```python
from build123d import *

# Parameters (mm, degrees)
BOSS_EXTRUDE1_DEPTH      = 37.5
BOSS_EXTRUDE1_DEPTH_BACK = 37.5
SKETCH1_W                = 20
SKETCH1_H                = 10
SKETCH3_W                = 20
SKETCH3_H                = 5
BOSS_EXTRUDE2_DEPTH      = 20
FILLET1_R                = 10
SKETCH4_R                = 2.75
CUT_EXTRUDE1_DEPTH       = 59.84301148
FILLET1_OF_MIRROR3_R     = 10
CHAMFER1_SIZE            = 8.660254038
CHAMFER1_SIZE_2          = 5
SKETCH6_R                = 8.5
CUT_EXTRUDE2_DEPTH       = 5
CUT_EXTRUDE3_DEPTH       = 59.576872569
CUT_EXTRUDE3_DEPTH_BACK  = 59.576872569
SKETCH7_R                = 2


# Some blends are built 0.0001 mm under size
with BuildPart() as part:
    # Sketch1 → Boss-Extrude1 (new, two sides: drawn at the far end of the back side and taken through both)
    with BuildSketch(Plane.XY.offset(-BOSS_EXTRUDE1_DEPTH_BACK)):
        Rectangle(SKETCH1_W, SKETCH1_H)
    extrude(amount=BOSS_EXTRUDE1_DEPTH + BOSS_EXTRUDE1_DEPTH_BACK)

    # Sketch3 → Boss-Extrude2 (add)
    with BuildSketch(Plane(origin=(0, 0, -37.5), x_dir=(-1, 0, 0), z_dir=(0, 0, -1))):
        Rectangle(SKETCH3_W, SKETCH3_H)
    boss_extrude2 = extrude(amount=BOSS_EXTRUDE2_DEPTH)

    # Fillet1
    fillet1_edges = [part.edges().sort_by_distance(p)[0] for p in [
        (-10, 0, -57.5),
        (10, 0, -57.5),
    ]]
    fillet(fillet1_edges, radius=FILLET1_R - 0.0001)  # a hair under: the kernel refuses the full size

    # Sketch4 → Cut-Extrude1 (cut, through all)
    with BuildSketch(Plane(origin=(0, 2.5, 0), x_dir=(1, 0, 0), z_dir=(0, 1, 0))):
        with Locations(Location((0, 47.5, 0), (0, 0, 270))):
            Circle(SKETCH4_R)
    cut_extrude1 = extrude(amount=-CUT_EXTRUDE1_DEPTH, mode=Mode.SUBTRACT)

    # Mirror3: Boss-Extrude2, Cut-Extrude1 across plane
    add(boss_extrude2.mirror(Plane.XY))
    add(cut_extrude1.mirror(Plane.XY), mode=Mode.SUBTRACT)

    # Fillet1 of Mirror3
    fillet1_of_mirror3_edges = [part.edges().sort_by_distance(p)[0] for p in [
        (-10, 0, 57.5),
        (10, 0, 57.5),
    ]]
    fillet(fillet1_of_mirror3_edges, radius=FILLET1_OF_MIRROR3_R - 0.0001)  # a hair under: the kernel refuses the full size

    # Chamfer1
    # the kernel refuses this chamfer: 8.660254038, 5 mm, written as the material it takes off along each edge
    with BuildSketch(Plane(origin=(32.404819853, 5, -37.5), x_dir=(0, 0.019326765612700598, 0.9998132206222078), z_dir=(-1, 0, 0))) as chamfer1_piece_1_section:
        Polygon((CHAMFER1_SIZE * 0.999813220604, -CHAMFER1_SIZE * 0.0193267656124), (-CHAMFER1_SIZE_2 * 0.0193267656127, -CHAMFER1_SIZE_2 * 0.999813220622), (0, 0), align=None)
    chamfer1_piece_1 = extrude(amount=64.809639706, mode=Mode.PRIVATE)
    chamfer1_piece_1 = split(chamfer1_piece_1, bisect_by=Plane(origin=(0, 2.5, -34.039331058), z_dir=(0, 1, 0)), keep=Keep.TOP, mode=Mode.PRIVATE)
    add(chamfer1_piece_1, mode=Mode.SUBTRACT)
    with BuildSketch(Plane(origin=(-32.404819853, -5, -37.5), x_dir=(0, -0.019326765612700598, 0.9998132206222078), z_dir=(1, 0, 0))) as chamfer1_piece_2_section:
        Polygon((CHAMFER1_SIZE * 0.999813220604, -CHAMFER1_SIZE * 0.0193267656124), (-CHAMFER1_SIZE_2 * 0.0193267656127, -CHAMFER1_SIZE_2 * 0.999813220622), (0, 0), align=None)
    chamfer1_piece_2 = extrude(amount=64.809639706, mode=Mode.PRIVATE)
    chamfer1_piece_2 = split(chamfer1_piece_2, bisect_by=Plane(origin=(0, -2.5, -34.039331058), z_dir=(0, -1, 0)), keep=Keep.TOP, mode=Mode.PRIVATE)
    add(chamfer1_piece_2, mode=Mode.SUBTRACT)
    with BuildSketch(Plane(origin=(-32.404819853, -5, 37.5), x_dir=(0, 0.999813220622208, 0.019326765612700494), z_dir=(1, 0, 0))) as chamfer1_piece_3_section:
        Polygon((CHAMFER1_SIZE * 0.999813220604, -CHAMFER1_SIZE * 0.0193267656124), (-CHAMFER1_SIZE_2 * 0.0193267656127, -CHAMFER1_SIZE_2 * 0.999813220622), (0, 0), align=None)
    chamfer1_piece_3 = extrude(amount=64.809639706, mode=Mode.PRIVATE)
    chamfer1_piece_3 = split(chamfer1_piece_3, bisect_by=Plane(origin=(0, 2.5, 37.476500167), z_dir=(0, 1, 0)), keep=Keep.TOP, mode=Mode.PRIVATE)
    add(chamfer1_piece_3, mode=Mode.SUBTRACT)
    with BuildSketch(Plane(origin=(-32.404819853, -5, 37.5), x_dir=(0, 0.999813220622208, 0.019326765612700494), z_dir=(1, 0, 0))) as chamfer1_piece_4_section:
        Polygon((CHAMFER1_SIZE * 0.999813220604, -CHAMFER1_SIZE * 0.0193267656124), (-CHAMFER1_SIZE_2 * 0.0193267656127, -CHAMFER1_SIZE_2 * 0.999813220622), (0, 0), align=None)
    chamfer1_piece_4 = extrude(amount=64.809639706, mode=Mode.PRIVATE)
    chamfer1_piece_4 = split(chamfer1_piece_4, bisect_by=Plane(origin=(0, -2.5, 35.327003025), z_dir=(0, -1, 0)), keep=Keep.TOP, mode=Mode.PRIVATE)
    add(chamfer1_piece_4, mode=Mode.SUBTRACT)
    with BuildSketch(Plane(origin=(32.404819853, 5, 37.5), x_dir=(0, -0.999813220622208, 0.019326765612700494), z_dir=(-1, 0, 0))) as chamfer1_piece_5_section:
        Polygon((CHAMFER1_SIZE * 0.999813220604, -CHAMFER1_SIZE * 0.0193267656124), (-CHAMFER1_SIZE_2 * 0.0193267656127, -CHAMFER1_SIZE_2 * 0.999813220622), (0, 0), align=None)
    chamfer1_piece_5 = extrude(amount=64.809639706, mode=Mode.PRIVATE)
    chamfer1_piece_5 = split(chamfer1_piece_5, bisect_by=Plane(origin=(0, -2.5, 37.476500167), z_dir=(0, -1, 0)), keep=Keep.TOP, mode=Mode.PRIVATE)
    add(chamfer1_piece_5, mode=Mode.SUBTRACT)
    with BuildSketch(Plane(origin=(32.404819853, 5, 37.5), x_dir=(0, -0.999813220622208, 0.019326765612700494), z_dir=(-1, 0, 0))) as chamfer1_piece_6_section:
        Polygon((CHAMFER1_SIZE * 0.999813220604, -CHAMFER1_SIZE * 0.0193267656124), (-CHAMFER1_SIZE_2 * 0.0193267656127, -CHAMFER1_SIZE_2 * 0.999813220622), (0, 0), align=None)
    chamfer1_piece_6 = extrude(amount=64.809639706, mode=Mode.PRIVATE)
    chamfer1_piece_6 = split(chamfer1_piece_6, bisect_by=Plane(origin=(0, 2.5, 35.327003025), z_dir=(0, 1, 0)), keep=Keep.TOP, mode=Mode.PRIVATE)
    add(chamfer1_piece_6, mode=Mode.SUBTRACT)

    # Sketch6 → Cut-Extrude2 (cut)
    with BuildSketch(Plane(origin=(0, 5, 0), x_dir=(1, 0, 0), z_dir=(0, 1, 0))):
        with Locations(Location((0, 0, 0), (0, 0, 270))):
            Circle(SKETCH6_R)
    extrude(amount=-CUT_EXTRUDE2_DEPTH, mode=Mode.SUBTRACT)

    # Sketch7 → Cut-Extrude3 (cut, two sides: drawn at the far end of the back side and taken through both)
    with BuildSketch(Plane(origin=(0, 0, 0), x_dir=(1, 0, 0), z_dir=(0, 1, 0)).offset(-CUT_EXTRUDE3_DEPTH_BACK)):
        with Locations(Location((0, 0, 0), (0, 0, 270))):
            Circle(SKETCH7_R)
    extrude(amount=CUT_EXTRUDE3_DEPTH + CUT_EXTRUDE3_DEPTH_BACK, mode=Mode.SUBTRACT)


solid = part.part
```
CAD build for the part. Positions are in the model's coordinates, mm. A direction names the side the tool comes from. Round coordinates to 2 decimals unless told otherwise and drop trailing zeros. Order: outer loops, then holes, each group sorted by start corner. A loop starts at its lowest first (then second) coordinate and runs counter-clockwise, first axis right, second up.
Q1. Slice it at D-D (y = 3.75). Write the cut outline in (x, z).
Q2. Which spindle directions (+Z, -Z, +X, -X, +Y, -Y) get a long thin tool onto all of the face, cutting with end or side? Do faces 5 (the flat face through (0, -2.5, -42)), 6 (the flat face through (0, 2.5, 43)), 7 (the cylindrical face through (8.428, 2.535, -1.107)), 8 (the cylindrical face through (-7.15, 0.04, -54.49)), 9 (the flat face through (0, 2.5, -42)). Say none if no direction does.
Q3. Slice it at A-A (z = 0). Write the cut outline in (x, y), and give its area (3 significant figures).
Q4. Slice it at C-C (x = -5.25). Write the cut outline in (y, z).
Q5. Drop flat-ended pins along their axis: pin 1 (1 mm diameter, centred on x = 0.5, z = -36, fed in from +Y); pin 2 (10 mm diameter, centred on x = 1, z = 45.5, fed in from -Y); pin 3 (6.5 mm diameter, centred on x = 0, z = 0, fed in from +Y). Give the stop position or say it passes through.
Q6. Slice it at B-B (y = -1). State how many separate pieces and enclosed holes the cut face has, and give its area (3 significant figures).
Q7. Wall check: L1, parallel to Z at x = -0.75, y = -2.25; L2, parallel to Z at x = 2.5, y = -1.75; L3, parallel to X at y = 0.3, z = 47.5. Give the ranges that are in metal, low to high.
Q8. Two-plate mould, pull along Z, no slides. Class faces 1 (the cylindrical face through (0.121, 0.035, -50.247)), 2 (the flat face through (2, -5, 1)), 3 (the flat face through (-0.14, -3.733, 33.232)), 4 (the cylindrical face through (-2, -3, 0)): pulls with the +Z half, pulls with the -Z half, needs draft (parallel to the pull), parting line crosses it, or undercut.
Results below:
1. outline: (-10, -31) - (10, -31) - (10, 33.22) - (-10, 33.22) - close; hole circle Ø17 at (0, 0)
2. face 5: -Z, +X, -X, -Y
2. face 6: +Z, +X, -X, +Y
2. face 7: +Y
2. face 8: -Z, -X, +Y, -Y
2. face 9: -Z, +X, -X, +Y
3. outline: (-10, -5) - (-2, -5) - (-2, 0) - (-8.5, 0) - (-8.5, 5) - (-10, 5) - close; (2, -5) - (10, -5) - (10, 5) - (8.5, 5) - (8.5, 0) - (2, 0) - close
3. area: 95.0 mm2
4. outline: (-5, -28.84) - (-2.5, -33.17) - (-2.5, -56.01) - (2.5, -56.01) - (2.5, -33.17) - (5, -28.84) - (5, -6.68) - (0, -6.68) - (0, 6.68) - (5, 6.68) - (5, 32.5) - (2.5, 33.94) - (2.5, 56.01) - (-2.5, 56.01) - (-2.5, 33.94) - (-5, 32.5) - close
5. pin 1: stops at y = 2.5
5. pin 2: stops at y = -2.5
5. pin 3: stops at y = 0
6. separate pieces: 1
6. enclosed holes: 3
6. area: 2,150 mm2
7. L1: z = -57.47 to -50.15, -44.85 to -1.85, 1.85 to 44.85, 50.15 to 57.47
7. L2: z = -57.18 to -48.65, -46.35 to 46.35, 48.65 to 57.18
7. L3: x = -10 to -2.75, 2.75 to 10
8. face 1: undercut
8. face 2: needs draft
8. face 3: pulls with the +Z half
8. face 4: undercut
